Part print with two shaded views. Sizes in mm from the minimum x, y, z corner. A direction names the side the tool comes from. Coordinates: 2 decimals unless noted, no trailing zeros. Order: outer loops, then holes, each group sorted by start corner. A loop starts at its lowest first (then second) coordinate and runs counter-clockwise, first axis right, second up. Notation, with made-up numbers: (30.25, 0) - (37.25, 0) arc R28 cw to (37.25, 27) - close; hole circle Ø3 at (-39.5, 74). An arc over 180 degrees is marked (long way). Return JSON: item names as keys, results as strings.
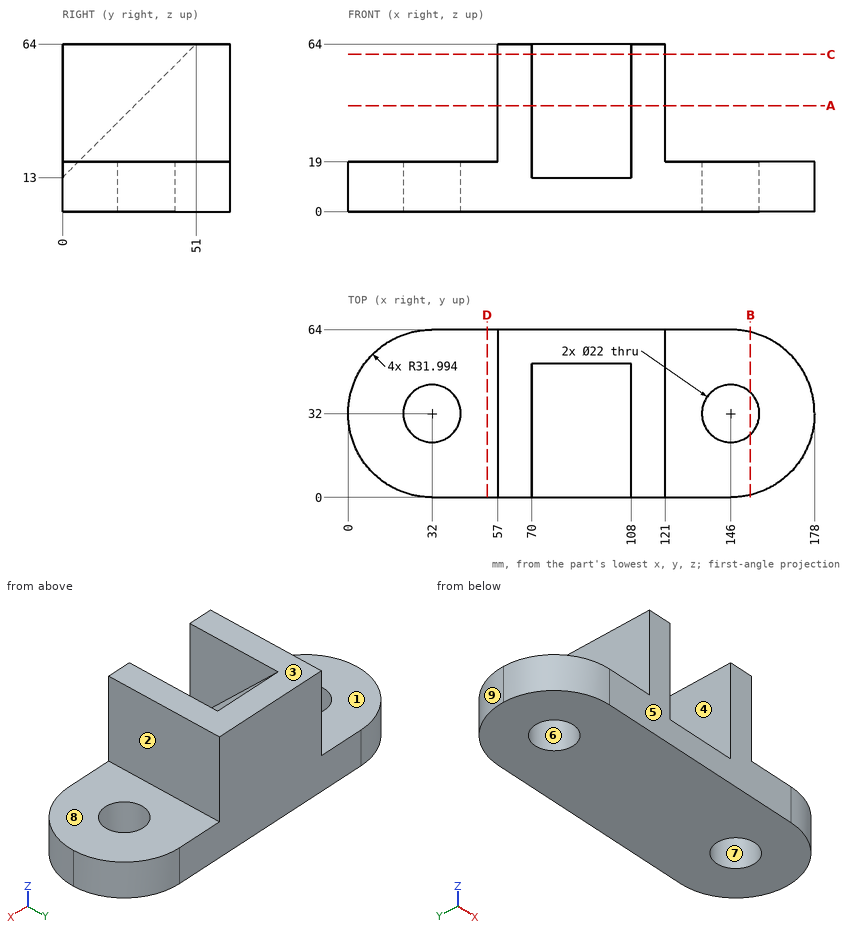
Item 1: Mould opens along Y. For the marked faces 6, 7, 8 and 9 say: released by +Y, released by -Y, zero draft, split by the parting line, or undercut.
Findings below:
{"face 6": "undercut", "face 7": "undercut", "face 8": "zero draft", "face 9": "released by +Y"}
Item 2: Band-saw the part on C-C, the plane z = 60. List the corners of the cut face in (x, y), then the cut area to 3 significant figures.
Findings below:
{"outline": "(57, 0) - (70, 0) - (70, 47) - (108, 47) - (108, 0) - (121, 0) - (121, 64) - (57, 64) - close", "area": "2,310 mm²"}
Item 3: Drop flat-ended pins along their axis: P1, Ø6, axis at y = 19.5, z = 52.5, coming from the +X side; P2, Ø20, axis at x = 146, y = 32, coming from the +Z side; P3, Ø4, axis at x = 48, y = 49.5, coming from the +Z side; P4, Ø12, axis at y = 17, z = 15, coming from the -X side. Give the stop position or say it passes through.
Findings below:
{"P1": "stops at x = 121", "P2": "passes through", "P3": "stops at z = 19", "P4": "stops at x = 1.29"}
Item 4: Wall check: L1, parallel to X at y = 32, z = 10; L2, parallel to X at y = 36, z = 53.5; L3, parallel to Y at x = 146, z = 10. Give the ranges that are in metal, low to high. Write a range as [from, to].
Findings below:
{"L1": "x = [0, 21], [43, 135], [157, 178]", "L2": "x = [57, 70], [108, 121]", "L3": "y = [0, 21], [43, 64]"}
Item 5: Band-saw the part on B-B, the plane x = 153.5. List the corners of the cut face in (y, z).
Findings below:
{"outline": "(0.89, 0) - (23.95, 0) - (23.95, 19) - (0.89, 19) - close; (40.05, 0) - (63.11, 0) - (63.11, 19) - (40.05, 19) - close"}
Item 6: Band-saw the part on A-A, the plane z = 40.5. List the corners of the cut face in (x, y).
Findings below:
{"outline": "(57, 0) - (70, 0) - (70, 27.5) - (108, 27.5) - (108, 0) - (121, 0) - (121, 64) - (57, 64) - close"}
Item 7: Which spindle directions (+Z, -Z, +X, -X, +Y, -Y) get a long thin tool onto all of the face, cutting with end or side? Do the marked faces 1, 2, 3, 4 and 5. Say none if no direction does.
Findings below:
{"face 1": "+Z, -X, +Y, -Y", "face 2": "+Z, +X, +Y, -Y", "face 3": "+Z, +X, -X, +Y, -Y", "face 4": "+Z, -Y", "face 5": "+Z, -Z, +X, -X, -Y"}
Item 8: Band-saw the part on D-D, the plane x = 53. List the corners of the cut face in (y, z), then the cut area to 3 significant figures.
Findings below:
{"outline": "(0, 0) - (64, 0) - (64, 19) - (0, 19) - close", "area": "1,220 mm²"}
